Verification items for the finished model (mm, model axes). Round coordinates to 2 decimals unless told otherwise and drop trailing zeros. Write each loop counter-clockwise with the first axis right and the second up, starting at its lowest first coordinate (ties: lowest second). Pieces come first, ordered by that corner, then holes. Notation, with made-up numbers: (85.5, 5.5) -> (108.5, 5.5) arc R7 cw to (108.5, 16.5) -> close; hole circle Ø5 at (39, 68.5). An arc over 180 degrees is marked (long way). Use CSV: the item, a comma, the result in double quotes.
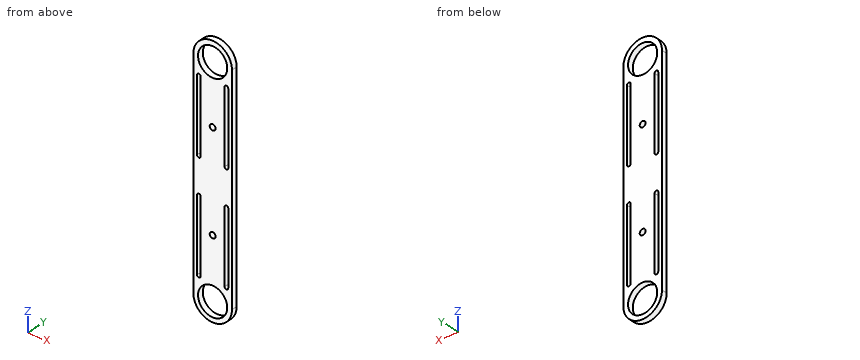
```python
from build123d import *

# Parameters (mm, degrees)
BOSS_EXTRUDE1_DEPTH     = 3.175
CUT_EXTRUDE2_DEPTH      = 131.960225355
CUT_EXTRUDE2_DEPTH_BACK = 131.960225355
CUT_EXTRUDE3_DEPTH      = 131.960225355
CUT_EXTRUDE3_DEPTH_BACK = 131.960225355
SKETCH4_R               = 1.6
CUT_EXTRUDE4_DEPTH      = 131.960225355
CUT_EXTRUDE4_DEPTH_BACK = 131.960225355
SKETCH5_R               = 7.95


with BuildPart() as part:
    # Sketch1 → Boss-Extrude1 (new body)
    with BuildSketch(Plane(origin=(0, 0, 0), x_dir=(1, 0, 0), z_dir=(0, 1, 0))):
        with BuildLine():
            Line((-10.5, 0), (-10.5, -120))
            ThreePointArc((-10.5, -120), (0, -130.5), (10.5, -120))
            Line((10.5, -120), (10.5, 0))
            ThreePointArc((10.5, 0), (0, 10.5), (-10.5, 0))
        make_face()
    extrude(amount=BOSS_EXTRUDE1_DEPTH)

    # Sketch3 → Cut-Extrude2 (cut, two sides: drawn at the far end of the back side and taken through both)
    with BuildSketch(Plane.XZ.offset(-CUT_EXTRUDE2_DEPTH_BACK)):
        with BuildLine():
            Line((-8.5, 110), (-8.5, 70))
            ThreePointArc((-8.5, 70), (-7.5, 69), (-6.5, 70))
            Line((-6.5, 70), (-6.5, 110))
            ThreePointArc((-6.5, 110), (-7.5, 111), (-8.5, 110))
        make_face()
        with BuildLine():
            Line((6.5, 110), (6.5, 70))
            ThreePointArc((6.5, 70), (7.5, 69), (8.5, 70))
            Line((8.5, 70), (8.5, 110))
            ThreePointArc((8.5, 110), (7.5, 111), (6.5, 110))
        make_face()
        with BuildLine():
            Line((8.5, 10), (8.5, 50))
            ThreePointArc((8.5, 50), (7.5, 51), (6.5, 50))
            Line((6.5, 50), (6.5, 10))
            ThreePointArc((6.5, 10), (7.5, 9), (8.5, 10))
        make_face()
        with BuildLine():
            Line((-8.5, 50), (-8.5, 10))
            ThreePointArc((-8.5, 10), (-7.5, 9), (-6.5, 10))
            Line((-6.5, 10), (-6.5, 50))
            ThreePointArc((-6.5, 50), (-7.5, 51), (-8.5, 50))
        make_face()
    extrude(amount=CUT_EXTRUDE2_DEPTH + CUT_EXTRUDE2_DEPTH_BACK, mode=Mode.SUBTRACT)

    # Sketch4 → Cut-Extrude3 (cut, two sides: drawn at the far end of the back side and taken through both)
    with BuildSketch(Plane(origin=(0, 3.175, 0), x_dir=(1, 0, 0), z_dir=(0, 1, 0)).offset(-CUT_EXTRUDE3_DEPTH_BACK)):
        with Locations(Location((0, -33.15, 0), (0, 0, 270))):
            Circle(SKETCH4_R)
        with Locations(Location((0, -87.15, 0), (0, 0, 270))):
            Circle(SKETCH4_R)
    extrude(amount=CUT_EXTRUDE3_DEPTH + CUT_EXTRUDE3_DEPTH_BACK, mode=Mode.SUBTRACT)

    # Sketch5 → Cut-Extrude4 (cut, two sides: drawn at the far end of the back side and taken through both)
    with BuildSketch(Plane(origin=(0, 3.175, 0), x_dir=(1, 0, 0), z_dir=(0, 1, 0)).offset(-CUT_EXTRUDE4_DEPTH_BACK)):
        with Locations(Location((0, 0, 0), (0, 0, 270))):
            Circle(SKETCH5_R)
        with Locations(Location((-0.003223035, -119.850034657, 0), (0, 0, 270))):
            Circle(SKETCH5_R)
    extrude(amount=CUT_EXTRUDE4_DEPTH + CUT_EXTRUDE4_DEPTH_BACK, mode=Mode.SUBTRACT)


solid = part.part
```
Q1. Section check C-C (y = 0.65). State how many separate pieces and enclosed holes the cut face has, plus the area to 3 significant figures.
Filled in:
separate pieces,"1"
enclosed holes,"8"
area,"2,120 mm²"
Q2. Section check A-A (z = 90.5). Record the cut outline in (x, y) (3 decimals), plus the area to 3 significant figures.
Filled in:
outline,"(-10.5, 0) -> (-8.5, 0) -> (-8.5, 3.175) -> (-10.5, 3.175) -> close; (-6.5, 0) -> (6.5, 0) -> (6.5, 3.175) -> (-6.5, 3.175) -> close; (8.5, 0) -> (10.5, 0) -> (10.5, 3.175) -> (8.5, 3.175) -> close"
area,"54.0 mm²"
Q3. Go/stop test with a flat-tipped pin: P1, Ø1.5, axis at x = 4.5, y = 1, coming from the +Z side. Record where the tip stops, or that it passes through.
Filled in:
P1,"z = 129.81"
Q4. Section check B-B (x = -5). Record the cut outline in (y, z) (3 decimals), plus the area to 3 significant figures.
Filled in:
outline,"(0, -9.233) -> (3.175, -9.233) -> (3.175, -6.181) -> (0, -6.181) -> close; (0, 6.181) -> (3.175, 6.181) -> (3.175, 113.667) -> (0, 113.667) -> close; (0, 126.033) -> (3.175, 126.033) -> (3.175, 129.233) -> (0, 129.233) -> close"
area,"361 mm²"
Q5. Material ranges on L1, parallel to X at y = 2.75, z = 109; L2, parallel to X at y = 1.75, z = 33.15; L3, parallel to Z at x = -6, y = 2.1, recorded low to high.
Filled in:
L1,"-10.5 to -8.5, -6.5 to 6.5, 8.5 to 10.5"
L2,"-10.5 to -8.5, -6.5 to -1.6, 1.6 to 6.5, 8.5 to 10.5"
L3,"-8.62 to -5.22, 5.22 to 114.63, 125.07 to 128.62"
